Autodesk Inventor part; units mm, degrees
ref_plane "YZ Plane" through (0, 0, 0) normal (1, 0, 0) x (0, 1, 0)
ref_plane "XZ Plane" through (0, 0, 0) normal (0, 1, 0) x (-1, 0, 0)
ref_plane "XY Plane" through (0, 0, 0) normal (0, 0, 1) x (1, 0, 0)
sketch "Sketch1" plane through (0, 0, 0) normal (0, 0, 1) x (1, 0, 0)
  circle A0 centre (0, 0) radius 161.1312
  circle A1 centre (0, 0) radius 151.6062
  circle A2 centre (0, 0) radius 153.1937
  circle A3 centre (0, 0) radius 159.5438
  dimension "d2" = 9.525
  dimension "d3" = 303.2125
  dimension "d4" = 322.2625
  dimension "d13" = 306.3875
  dimension "d14" = 319.0875
  dimension "d15" = 6.35
  dimension "d16" = 1.5875
  dimension "d35" = 0
extrude "Extrusion1" add sketch "Sketch1" along normal blind 1136.65 contours A3
sketch "Sketch2" plane through (0, 0, 0) normal (1, 0, 0) x (0, 1, 0)
  circle A0 centre (0, 914.4) radius 25.4
  line L0 (159.5438, 1136.65) -> (-159.5438, 1136.65)
  circle A1 centre (0, 1025.525) radius 3.175
  circle A2 centre (42.8625, 939.8) radius 3.175
  circle A3 centre (-42.8625, 939.8) radius 3.175
  circle A4 centre (42.8532, 889) radius 3.175
  circle A5 centre (-42.8718, 889) radius 3.175
  point P0 (0, 0)
  point P1 (0, 1136.65)
  dimension "d21" = 50.8
  dimension "d22" = 222.25
  dimension "d23" = 6.35
  dimension "d24" = 111.125
  dimension "d25" = 6.35
  dimension "d26" = 6.35
  dimension "d27" = 85.725
  dimension "d28" = 42.8625
  dimension "d29" = 6.35
  dimension "d30" = 6.35
  dimension "d31" = 85.725
  dimension "d32" = 50.8
extrude "Extrusion3" cut sketch "Sketch2" along normal through all
properties part number "tube"
Input: part model. Units: mm. Frame: model coordinates. Give positions to 0.01 mm unless a question says otherwise; leave off trailing zeros. Order: outer loops, then holes, each group sorted by start corner. A loop starts at its lowest first (then second) coordinate and runs counter-clockwise, first axis right, second up. Notation, with made-up numbers: (-18, 71.5) - (-3, 71.5) arc R13 cw to (-3, 92.5) - close; hole circle Ø6 at (-19.5, -12.75). An arc over 180 degrees is marked (long way). Put each result on its own line as item: value.
Item 1: Section query D-D, the plane z = 914.4. Return loops of the section in (x, y).
Found:
outline: (151.07, -25.4) arc R153.19 cw (long way) to (151.07, 25.4) - (157.51, 25.4) arc R159.54 ccw (long way) to (157.51, -25.4) - close
Item 2: Section query A-A, the plane x = 0. Return loops of the section in (y, z).
Found:
outline: (-159.54, 0) - (-153.19, 0) - (-153.19, 1136.65) - (-159.54, 1136.65) - close; (153.19, 0) - (159.54, 0) - (159.54, 1136.65) - (153.19, 1136.65) - close
Item 3: Section query C-C, the plane z = 642. Return loops of the section in (x, y).
Found:
outline: circle Ø319.09 at (0, 0); hole circle Ø306.39 at (0, 0)
Item 4: Draft query along Y for faces 1 (the cylindrical face through (155.249, -5.506, 939.196)), 2 (the cylindrical face through (-34.59, 155.75, 560.37)), 3 (the cylindrical face through (-121.569, 93.216, 560.368)), 4 (the flat face through (-60, 143, 0)). Return one class per face: +Y half, -Y half, draft (parallel to the pull), parting line (faces both ways), or undercut.
Found:
face 1: undercut
face 2: parting line
face 3: undercut
face 4: draft
Item 5: Section query B-B, the plane y = -97. Return loops of the section in (x, z).
Found:
outline: (-126.67, 0) - (-118.57, 0) - (-118.57, 1136.65) - (-126.67, 1136.65) - close; (118.57, 0) - (126.67, 0) - (126.67, 1136.65) - (118.57, 1136.65) - close
Item 6: Ray query, L1, parallel to X at y = -74, z = 91; L2, parallel to X at y = 10, z = 430.5; L3, parallel to Y at x = -35, z = 532. Return the intervals inside material, ascending. Write a range as from..to.
Found:
L1: x = -141.34..-134.14, 134.14..141.34
L2: x = -159.23..-152.87, 152.87..159.23
L3: y = -155.66..-149.14, 149.14..155.66
Item 7: Contact query for flat-ended pins moving along their axis: pin 1 (8 mm diameter, centred on y = 98.5, z = 346, fed in from +X); pin 2 (4 mm diameter, centred on x = -80.5, z = 248.5, fed in from +Y); pin 3 (12 mm diameter, centred on y = -112, z = 545, fed in from -X). Output: stop coordinate, or through.
Found:
pin 1: stops at x = 128.55
pin 2: stops at y = 138.9
pin 3: stops at x = -119.24
